Can you work these out from the model? Positions are in its coordinate system, mm. Face numbers are marked on the shaded views. Coordinates: 2 decimals unless noted, no trailing zeros. Write each loop counter-clockwise with the first axis right and the second up, starting at its lowest first coordinate (ties: lowest second). Pieces come first, ordered by that corner, then holes. Notation, with made-up numbers: M 29.25,28 L 87.25,28 A14 cw 87.25,46 Z; hole C 51.25,-5 d6. An arc over 180 degrees is marked long. Answer as a JSON object with one key per item and string values. Group by question number.
from build123d import *

# Parameters (mm, degrees)
CUT_EXTRUDE1_DEPTH                               = 56.357926262
SKETCH3_W                                        = 10
SKETCH3_H                                        = 6
CBORE_START                                      = -35.263917504
CBORE_FOR_M2_HEX_HEAD_MACHINE_SCREW1_OUT_R       = 2
CBORE_FOR_M2_HEX_HEAD_MACHINE_SCREW1_DEPTH       = 23.263917504
CBORE_START_2                                    = -12
CBORE_FOR_M2_HEX_HEAD_MACHINE_SCREW1_2_O_R       = 1.2295
CBORE_FOR_M2_HEX_HEAD_MACHINE_SCREW1_2_DEPTH     = 6.12732314
CBORE_FOR_M2_HEX_HEAD_MACHINE_SCREW2_D           = 2.459
CBORE_FOR_M2_HEX_HEAD_MACHINE_SCREW2_DEPTH       = 27.463932023
CBORE_FOR_M2_HEX_HEAD_MACHINE_SCREW2_CBORE_D     = 4
CBORE_FOR_M2_HEX_HEAD_MACHINE_SCREW2_CBORE_DEPTH = 23.263932023
CHAMFER1_SIZE                                    = 0.2705
FILLET1_R                                        = 0.2


# Read off the part's stored shape, not the designer's step: CBORE for M2 Hex Head Machine Screw1
with BuildPart() as part:
    # Sketch1 → Revolve1 (revolve)
    with BuildSketch(Plane(origin=(0, 0, 0), x_dir=(-1, 0, 0), z_dir=(0, 0, -1)), mode=Mode.PRIVATE) as revolve1_sk:
        with BuildLine():
            Line((-5, 38.5), (-5, 0))
            Line((-5, 0), (5, 0))
            Line((5, 0), (5, 38.5))
            Line((5, 38.5), (3.968118785, 38.5))
            Line((3.968118785, 38.5), (2.850084796, 36.563508327))
            ThreePointArc((2.850084796, 36.563508327), (0, 34.5), (-2.850084796, 36.563508327))
            Line((-2.850084796, 36.563508327), (-3.968118785, 38.5))
            Line((-3.968118785, 38.5), (-5, 38.5))
        make_face()
    revolve(revolve1_sk.sketch.rotate(Axis((5, 0, 0), (-1, 0, 0)), 180), axis=Axis((5, 0, 0), (-1, 0, 0)))

    # Sketch2 → Cut-Extrude1 (cut, through all)
    with BuildSketch(Plane.ZY.offset(5)):
        with BuildLine():
            Line((2, 5.656854249), (2, 7.8))
            Line((2, 7.8), (-2, 7.8))
            Line((-2, 7.8), (-2, 5.656854249))
            ThreePointArc((-2, 5.656854249), (0, 6), (2, 5.656854249))
        make_face()
    extrude(amount=-CUT_EXTRUDE1_DEPTH, mode=Mode.SUBTRACT)

    # Sketch3 → Cut-Revolve1 (revolve, cut)
    with BuildSketch(Plane(origin=(0, 0, 0), x_dir=(-1, 0, 0), z_dir=(0, 0, -1)), mode=Mode.PRIVATE) as cut_revolve1_sk:
        with Locations((0, 3)):
            Rectangle(SKETCH3_W, SKETCH3_H)
    revolve(cut_revolve1_sk.sketch.rotate(Axis((5, 0, 0), (-1, 0, 0)), 180), axis=Axis((5, 0, 0), (-1, 0, 0)), mode=Mode.SUBTRACT)

    # CBORE for M2 Hex Head Machine Screw1 out → CBORE for M2 Hex Head Machine Screw1 (cut)
    with BuildSketch(Plane.XY.offset(CBORE_START)):
        Circle(CBORE_FOR_M2_HEX_HEAD_MACHINE_SCREW1_OUT_R)
    extrude(amount=CBORE_FOR_M2_HEX_HEAD_MACHINE_SCREW1_DEPTH, mode=Mode.SUBTRACT)

    # CBORE for M2 Hex Head Machine Screw1 2 o → CBORE for M2 Hex Head Machine Screw1 2 (cut)
    with BuildSketch(Plane.XY.offset(CBORE_START_2)):
        Circle(CBORE_FOR_M2_HEX_HEAD_MACHINE_SCREW1_2_O_R)
    extrude(amount=CBORE_FOR_M2_HEX_HEAD_MACHINE_SCREW1_2_DEPTH, mode=Mode.SUBTRACT)

    # CBORE for M2 Hex Head Machine Screw2
    with Locations(Plane(origin=(0, 35.263932023, 0), x_dir=(1, 0, 0), z_dir=(0, 1, 0))):
        with Locations((0, 0)):
            CounterBoreHole(CBORE_FOR_M2_HEX_HEAD_MACHINE_SCREW2_D / 2, CBORE_FOR_M2_HEX_HEAD_MACHINE_SCREW2_CBORE_D / 2, CBORE_FOR_M2_HEX_HEAD_MACHINE_SCREW2_CBORE_DEPTH, depth=CBORE_FOR_M2_HEX_HEAD_MACHINE_SCREW2_DEPTH)

    # Chamfer1
    chamfer1_edges = [part.edges().sort_by_distance(p)[0] for p in [
        (-1.2295, 0, -12),
        (1.2295, 12, 0),
    ]]
    chamfer(chamfer1_edges, length=CHAMFER1_SIZE)

    # Fillet1
    fillet1_edges = [part.edges().sort_by_distance(p)[0] for p in [
        (0, 7.8, -2),
        (0, 7.8, 2),
    ]]
    fillet(fillet1_edges, radius=FILLET1_R)


solid = part.part
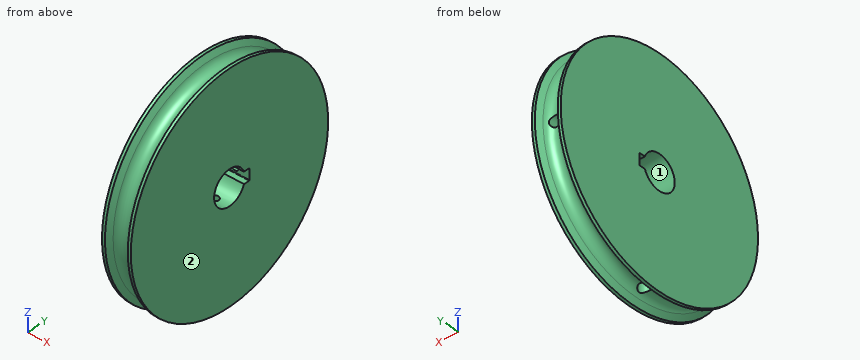
Q1. Will these pins go through, and if not, where does the flat tip stop? pin 1 (3 mm diameter, centred on x = -1, z = -0.5, fed in from +Y); pin 2 (4.5 mm diameter, centred on x = 0, y = 0, fed in from -Z); pin 3 (4 mm diameter, centred on x = 0, y = 0, fed in from +Z); pin 4 (15.5 mm diameter, centred on y = 0, z = 0, fed in from -X).
Q2. Please list where these lines run through material, in increasing order: L1, parallel to X at y = 9.45, z = 0; L2, parallel to Z at x = -1.25, y = 21; L3, parallel to Z at x = -2.25, y = 3.
Q3. If we section it at B-B on x = 0: List the corners of the cut face in (y, z) for me, and give its area (3 significant figures).
Q4. We'd pull the mould along Y, two halves only. Please class the marked faces 1 and 2: pulls with the +Y half, pulls with the -Y half, needs draft (parallel to the pull), parting line crosses it, or undercut.
Q5. If we section it at A-A on z = 0: List the corners of the cut face in (x, y) for me, and give its area (3 significant figures).
Reply:
{
 "1": {"pin 1": "y = 35.84", "pin 2": "z = -35.52", "pin 3": "z = 35.26", "pin 4": "x = -5"},
 "2": {"L1": "-5 to -1.23, 1.23 to 5", "L2": "-27.72 to -1.56, 1.56 to 27.72", "L3": "-35.39 to -5.2, 5.2 to 35.39"},
 "3": {"outline": "M -2,-34.44 L -2,-12 L -1.5,-12 L -1.23,-11.73 L -1.23,-5.87 A6 cw long 5.66,2 L 7.6,2 A0.2 cw 7.8,1.8 L 7.8,1.23 L 11.73,1.23 L 12,1.5 L 12,2 L 34.44,2 A34.5 ccw long Z; M 1.23,-11.73 L 1.5,-12 L 2,-12 L 2,-34.44 A34.5 ccw 34.44,-2 L 12,-2 L 12,-1.5 L 11.73,-1.23 L 7.8,-1.23 L 7.8,-1.8 A0.2 cw 7.6,-2 L 5.66,-2 A6 cw 1.23,-5.87 Z", "area": "3,410 mm^2"},
 "4": {"face 1": "undercut", "face 2": "needs draft"},
 "5": {"outline": "M -5,-38.5 L -3.97,-38.5 L -2.85,-36.56 A3 cw 2.85,-36.56 L 3.97,-38.5 L 5,-38.5 L 5,-6 L -5,-6 Z; M -5,7.8 L -1.23,7.8 L -1.23,11.73 L -1.5,12 L -2,12 L -2,35.26 A3 cw -2.85,36.56 L -3.97,38.5 L -5,38.5 Z; M 1.23,7.8 L 5,7.8 L 5,38.5 L 3.97,38.5 L 2.85,36.56 A3 cw 2,35.26 L 2,12 L 1.5,12 L 1.23,11.73 Z", "area": "487 mm^2"}
}
